```python
from build123d import *

# Parameters (mm, degrees)
F0_W     = 78
F0_H     = 2
F0_W_2   = 2
F0_H_2   = 78
F1_DEPTH = 2


with BuildPart() as f1:
    # F0 (on Top) → F1 (new body)
    with BuildSketch(Plane.XY):
        with Locations((0, 48)):
            Rectangle(F0_W, F0_H)
        Polygon((47, 47), (39, 47), (-39, 47), (-47, 47), (-47, 39), (-47, -39), (-47, -47), (-39, -47), (39, -47), (47, -47), (47, -39), (47, 39), align=None)
        with Locations((48, 0)):
            Rectangle(F0_W_2, F0_H_2)
        with Locations((-48, 0)):
            Rectangle(F0_W_2, F0_H_2)
        with Locations((0, -48)):
            Rectangle(F0_W, F0_H)
    extrude(amount=F1_DEPTH)


solid = f1.part
```
For this review, take the finished solid that the model builds, in its own axes (mm). Round coordinates to 2 decimals unless told otherwise and drop trailing zeros. Write each loop counter-clockwise with the first axis right and the second up, starting at its lowest first coordinate (ties: lowest second). Pieces come first, ordered by that corner, then holes. Notation, with made-up numbers: (20, 28) -> (37, 28) arc R35 ccw to (37, 63) -> close; hole circle Ø9 at (88, -20.75). An arc over 180 degrees is marked (long way). Use one line per item in the form item = value.
Q1. Clearance check with flat-ended pins moving along their axes: pin 1 Ø0.6 at (x, z) = (43, 0.5) entering from -Y; pin 2 Ø1 at (y, z) = (42.5, 0.5) entering from -X; pin 3 Ø12 at (x, y) = (36.5, 7) entering from -Z; pin 4 Ø1 at (y, z) = (48, 1) entering from +X. State where each tip first meets the part, or that it passes through.
Resolved:
pin_1 = -47
pin_2 = -47
pin_3 = 0
pin_4 = 39
Q2. Consider section A-A (x = 41). State the section outline as (y, z) points.
Resolved:
outline = (-47, 0) -> (47, 0) -> (47, 2) -> (-47, 2) -> close
Q3. To check wall thickness, follow probe 1 along X at (y, z) = (-43, 1.35). State the ranges of the line that lie inside material, in increasing order. Write a range as from..to.
Resolved:
probe_1 = -47..47
